from build123d import *

# Parameters (mm, degrees)
SKETCH1_R                = 9.525
SKETCH1_R_2              = 4.7498
BOSS_EXTRUDE1_DEPTH      = 131.953
SKETCH2_R                = 8.9408
SKETCH2_R_2              = 4.7498
BOSS_EXTRUDE2_DEPTH      = 1.0668
SKETCH4_R                = 9.525
SKETCH4_R_2              = 4.7498
BOSS_EXTRUDE4_DEPTH      = 2.54
CHAMFER1_SIZE            = 0.762
CHAMFER1_OF_MIRROR1_SIZE = 0.762


with BuildPart() as part:
    # Sketch1 → Boss-Extrude1 (new, symmetric)
    with BuildSketch(Plane.XY):
        Circle(SKETCH1_R)
        Circle(SKETCH1_R_2, mode=Mode.SUBTRACT)
    extrude(amount=BOSS_EXTRUDE1_DEPTH, both=True)

    # Sketch2 → Boss-Extrude2 (add)
    with BuildSketch(Plane.XY.offset(131.953)):
        Circle(SKETCH2_R)
        Circle(SKETCH2_R_2, mode=Mode.SUBTRACT)
    boss_extrude2 = extrude(amount=BOSS_EXTRUDE2_DEPTH)

    # Sketch4 → Boss-Extrude4 (add)
    with BuildSketch(Plane.XY.offset(133.0198)):
        Circle(SKETCH4_R)
        Circle(SKETCH4_R_2, mode=Mode.SUBTRACT)
    boss_extrude4 = extrude(amount=BOSS_EXTRUDE4_DEPTH)

    # Chamfer1
    chamfer1_edges = [part.edges().sort_by_distance(p)[0] for p in [
        (-9.525, 0, 135.5598),
    ]]
    chamfer(chamfer1_edges, length=CHAMFER1_SIZE)

    # Mirror1: Boss-Extrude2, Boss-Extrude4 across plane
    add(boss_extrude2.mirror(Plane.XY))
    add(boss_extrude4.mirror(Plane.XY))

    # Chamfer1 of Mirror1
    chamfer1_of_mirror1_edges = [part.edges().sort_by_distance(p)[0] for p in [
        (-9.525, 0, -135.5598),
    ]]
    chamfer(chamfer1_of_mirror1_edges, length=CHAMFER1_OF_MIRROR1_SIZE)


solid = part.part
Source: CAD feature listing. Evaluate the final solid. Frame: model axes, mm. A direction names the side the tool comes from. Round coordinates to 2 decimals unless told otherwise and drop trailing zeros. Loops run counter-clockwise (first coordinate to the right, second up) from the corner with the lowest first, then second, coordinate; pieces in that order, holes last. Notation, with made-up numbers: (23, -13) -> (56, -13) arc R17 ccw to (56, 17) -> close; hole circle Ø1 at (-33.5, 74.5). An arc over 180 degrees is marked (long way). Answer as a JSON object with one key per item and string values. Group by question number.
Q1. Section query C-C (z = 39). Output: boundary loops of the cut face in (x, y) (3 decimals), plus the area to 3 significant figures.
Q2. Section query A-A (x = 0). Output: boundary loops of the cut face in (y, z) (3 decimals), plus the area to 3 significant figures.
Q3. Access query for faces 1 (the cylindrical face through (-3.5, 3.21, 1.9)), 2 (the flat face through (6, -7, 131.953)). Directions: +Z, -Z, +X, -X, +Y, -Y. A direction counts if a zero-diameter tool reaches every point of the face in a straight line with its end or side. Return the directions, or none.
Q4. Contact query for flat-ended pins moving along their axis: P1, Ø5, axis at x = -6, z = 21, coming from the +Y side; P2, Ø5, axis at x = -5, z = 43, coming from the +Y side; P3, Ø4, axis at y = -3, z = -70, coming from the +X side. Output: stop coordinate, or through.
Q5. Mould query, pull axis Z, two halves, no side actions, for faces 3 (the cylindrical face through (-7.559, -5.796, 1.847)), 4 (the flat face through (6, -7, -131.953)), 5 (the flat face through (4, -4, -135.56)), 6 (the flat face through (4, -4, 135.56)). Classes: pulls with the +Z half, pulls with the -Z half, needs draft (parallel to the pull), parting line crosses it, or undercut.
Q6. Ray query, line 1 (Y direction, x = 0, z = -53.5) (3 decimals); line 2 (X direction, y = 0.25, z = -108); line 3 (Y direction, x = 2.25, z = -57.5). Return the intervals inside material, ascending. Write a range as from..to.
Completed:
{
 "1": {"outline": "circle Ø19.05 at (0, 0); hole circle Ø9.5 at (0, 0)", "area": "214 mm²"},
 "2": {"outline": "(-9.525, -134.798) -> (-8.763, -135.56) -> (-4.75, -135.56) -> (-4.75, 135.56) -> (-8.763, 135.56) -> (-9.525, 134.798) -> (-9.525, 133.02) -> (-8.941, 133.02) -> (-8.941, 131.953) -> (-9.525, 131.953) -> (-9.525, -131.953) -> (-8.941, -131.953) -> (-8.941, -133.02) -> (-9.525, -133.02) -> close; (4.75, -135.56) -> (8.763, -135.56) -> (9.525, -134.798) -> (9.525, -133.02) -> (8.941, -133.02) -> (8.941, -131.953) -> (9.525, -131.953) -> (9.525, 131.953) -> (8.941, 131.953) -> (8.941, 133.02) -> (9.525, 133.02) -> (9.525, 134.798) -> (8.763, 135.56) -> (4.75, 135.56) -> close", "area": "2,590 mm²"},
 "3": {"face 1": "+Z, -Z", "face 2": "none"},
 "4": {"P1": "y = 8.86", "P2": "y = 9.19", "P3": "x = 9.47"},
 "5": {"face 3": "needs draft", "face 4": "undercut", "face 5": "pulls with the -Z half", "face 6": "pulls with the +Z half"},
 "6": {"line 1": "-9.525..-4.75, 4.75..9.525", "line 2": "-9.52..-4.74, 4.74..9.52", "line 3": "-9.26..-4.18, 4.18..9.26"}
}
